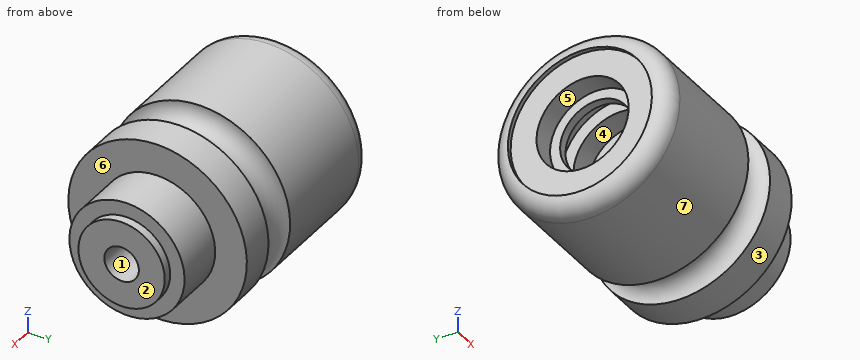
```python
from build123d import *

# Parameters (mm, degrees)
F4_R = 5.99999


# Not quite as in the source:
# - a fillet or chamfer is up to 0.001 mm smaller than in the source, because OpenCascade refuses the exact size


with BuildPart() as f1:
    # F0 (on Front) → F1 (revolve)
    with BuildSketch(Plane.XZ):
        with BuildLine():
            Line((0, 31), (0, 0))
            Line((0, 0), (88, 0))
            Line((88, 0), (88, 15))
            Line((88, 15), (85, 15))
            Line((85, 15), (85, 20))
            Line((85, 20), (68, 20))
            Line((68, 20), (68, 31))
            Line((68, 31), (56, 31))
            ThreePointArc((56, 31), (50, 25), (44, 31))
            Line((44, 31), (0, 31))
        make_face()
    revolve(axis=Axis((63.3454471827, 0, 0), (1, 0, 0)))

    # F2 (on Front) → F3 (revolve, cut)
    with BuildSketch(Plane.XZ):
        Polygon((0, 25), (0, 0), (88, 0), (88, 6), (30, 6), (30, 16), (22, 16), (22, 20.5), (12, 20.5), (12, 12.5), (9, 12.5), (9, 16), (1.5, 16), (1.5, 25), align=None)
    revolve(axis=Axis((-10.8097042758, 0, 0), (-1, 0, 0)), mode=Mode.SUBTRACT)

    # F4 (radius 6 in the source; OpenCascade refuses exactly that, so slightly less here)
    f4_edges = [f1.edges().sort_by_distance(p)[0] for p in [
        (0, 0, -31),
    ]]
    fillet(f4_edges, radius=F4_R)


solid = f1.part
```
Geometry check sheet. Reference: the model listing, model coordinates, mm. Face numbers are marked on the shaded views. A direction names the side the tool comes from. Give positions to 0.01 mm unless a question says otherwise; leave off trailing zeros. Order: outer loops, then holes, each group sorted by start corner. A loop starts at its lowest first (then second) coordinate and runs counter-clockwise, first axis right, second up.
1. Section check A-A, the plane x = 34.5. Enter the section's corners in (y, z).
2. Gauge pin test, flat ends, axial feed: pin 1 Ø2 at (y, z) = (-7, -8.5) entering from -X; pin 2 Ø1.5 at (x, y) = (11.5, 13) entering from +Z; pin 3 Ø8 at (x, y) = (71, -3) entering from -Z. Record the tip position at first contact, or that the pin passes through.
3. Release check for a two-part mould opening along Z. For the marked faces 1, 2, 3 and 4 record: pulls with the +Z half, pulls with the -Z half, needs draft (parallel to the pull), parting line crosses it, or undercut.
4. Thickness scan on L1, parallel to X at y = 0.5, z = -17; L2, parallel to X at y = 10, z = 11.5; L3, parallel to Y at x = 14.25, z = 0. Record the ranges inside material, lowest first.
5. Section check B-B, the plane x = 80.5. Enter the section's corners in (y, z), and give its area (3 significant figures).
6. Access from +Z, -Z, +X, -X, +Y, -Y to the whole of each face (thin tool, end or side, straight path). Record for the marked faces 5, 6 and 7.
Values follow:
1. outline: circle Ø62 at (0, 0); hole circle Ø12 at (0, 0)
2. pin 1: stops at x = 30
2. pin 2: stops at z = 28.48
2. pin 3: stops at z = -31
3. face 1: undercut
3. face 2: needs draft
3. face 3: parting line crosses it
3. face 4: undercut
4. L1: x = 1.5 to 12, 22 to 85
4. L2: x = 9 to 12, 30 to 85
4. L3: y = -31 to -20.5, 20.5 to 31
5. outline: circle Ø40 at (0, 0); hole circle Ø12 at (0, 0)
5. area: 1,140 mm2
6. face 5: -X
6. face 6: +X
6. face 7: +X, -X
